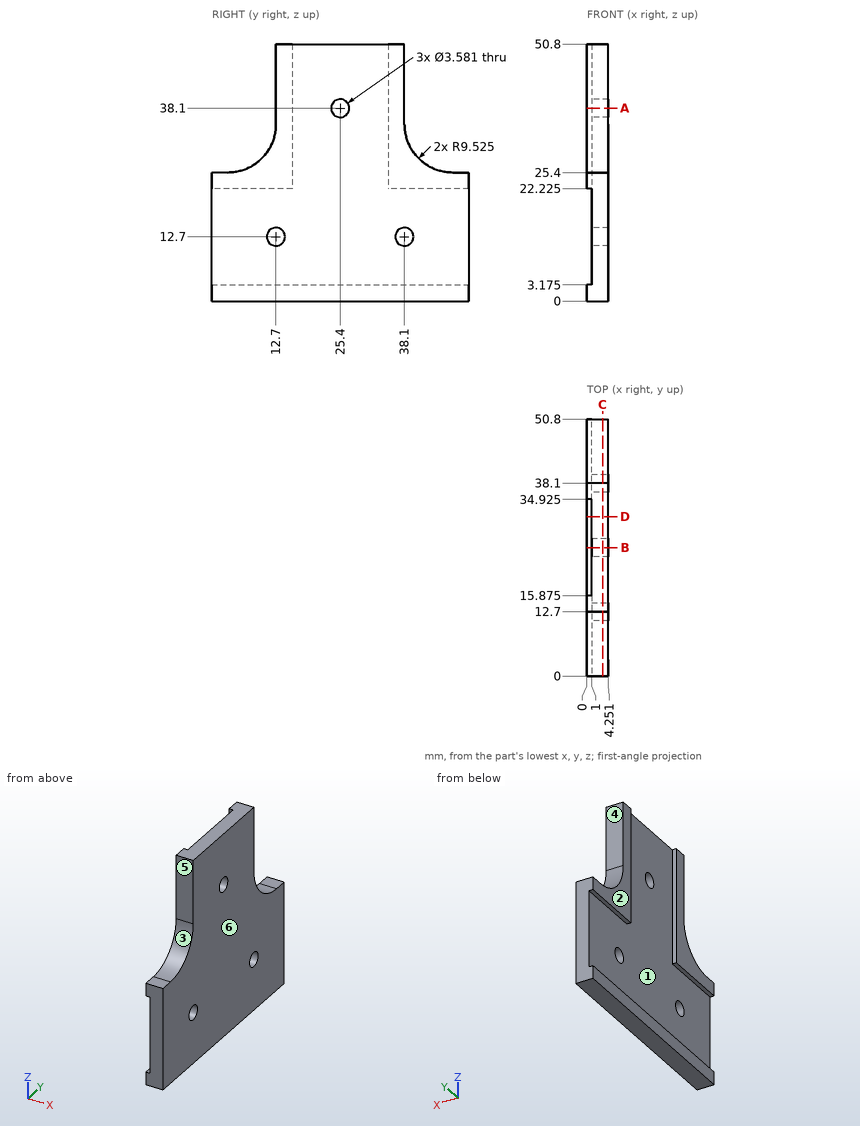
The figure shows three views and two pictorial views of one solid part (mm, origin at its lowest corner). Answer the questions. A direction names the side the tool comes from. Round coordinates to 2 decimals unless told otherwise and drop trailing zeros. Order: outer loops, then holes, each group sorted by start corner. A loop starts at its lowest first (then second) coordinate and runs counter-clockwise, first axis right, second up.
Q1. A cutting plane is placed at B-B, the plane y = 25.4. Determine the outline of the cut face in (x, z) (1 decimal), then the cut area to 3 significant figures.
Solution:
outline: (0, 0) - (4.3, 0) - (4.3, 36.3) - (1, 36.3) - (1, 3.2) - (0, 3.2) - close; (1, 39.9) - (4.3, 39.9) - (4.3, 50.8) - (1, 50.8) - close
area: 157 mm2
Q2. Find the intervals of material crossed by line 1 along Y through (x, z) = (2.2, 38.1); line 2 along Z through (x, y) = (3.55, 25.4); line 3 along X through (y, z) = (27.5, 47), in increasing order.
Solution:
line 1: y = 12.7 to 23.61, 27.19 to 38.1
line 2: z = 0 to 36.31, 39.89 to 50.8
line 3: x = 1 to 4.25
Q3. A cutting plane is placed at C-C, the plane x = 3.15. Count the separate pieces of the cut face and the enclosed holes in it, then the cut area to 3 significant figures.
Solution:
separate pieces: 1
enclosed holes: 3
area: 1,940 mm2
Q4. The mould has two halves that part along Z. Classify the marked faces 1, 2 and 3: pulls with the +Z half, pulls with the -Z half, needs draft (parallel to the pull), parting line crosses it, or undercut.
Solution:
face 1: undercut
face 2: needs draft
face 3: pulls with the +Z half
Q5. A tool of negligible diameter and unlimited length cuts with its end or side. For the marked faces 4, 5 and 6, from which of +Z, -Z, +X, -X, +Y, -Y can it reach the whole face along a straight path? Write none if from no direction.
Solution:
face 4: +Z, +X, -X, +Y
face 5: +Z, +X, -X, -Y
face 6: +Z, -Z, +X, +Y, -Y
Q6. A cutting plane is placed at A-A, the plane z = 38.1. Determine the outline of the cut face in (x, y) (1 decimal).
Solution:
outline: (0, 12.7) - (4.3, 12.7) - (4.3, 23.6) - (1, 23.6) - (1, 15.9) - (0, 15.9) - close; (0, 34.9) - (1, 34.9) - (1, 27.2) - (4.3, 27.2) - (4.3, 38.1) - (0, 38.1) - close
Q7. Given pin 1 Ø2.5 at (x, y) = (2, 49.5) entering from +Z; pin 2 Ø1.5 at (y, z) = (25.5, 6) entering from -X; pin 3 Ø0.5 at (x, y) = (0.5, 22) entering from +Z (3 decimals); pin 4 Ø1.5 at (x, z) = (1.5, 18) entering from -Y, each flat-ended and moving along its own axis, determine where each tip first touches the part or whether it passes through.
Solution:
pin 1: stops at z = 25.4
pin 2: stops at x = 1
pin 3: stops at z = 3.175
pin 4: stops at y = 0
Q8. A cutting plane is placed at D-D, the plane y = 31.5. Determine the outline of the cut face in (x, z) (1 decimal), then the cut area to 3 significant figures.
Solution:
outline: (0, 0) - (4.3, 0) - (4.3, 50.8) - (1, 50.8) - (1, 3.2) - (0, 3.2) - close
area: 168 mm2
